```python
from build123d import *

# Parameters (mm, degrees)
ESQUISSE1_R             = 20.5
ESQUISSE1_R_2           = 13
BOSS_EXTRU_1_DEPTH      = 4.5
ENL_V_MAT_EXTRU_1_REACH = 6.5
ESQUISSE2_R             = 1.5
ESQUISSE2_R_2           = 2.11
ENL_V_MAT_EXTRU_2_DEPTH = 2.5


with BuildPart() as part:
    # Esquisse1 → Boss.-Extru.1 (new body)
    with BuildSketch(Plane.XY):
        Circle(ESQUISSE1_R)
        Circle(ESQUISSE1_R_2, mode=Mode.SUBTRACT)
    extrude(amount=BOSS_EXTRU_1_DEPTH)

    # Esquisse2 → Enlèv. mat.-Extru.1 (cut, up to next)
    with BuildSketch(Plane.XY.offset(4.5), mode=Mode.PRIVATE) as enl_v_mat_extru_1_sk1:
        with Locations((0, 17.5)):
            Circle(ESQUISSE2_R)
    enl_v_mat_extru_1_tool1 = extrude(enl_v_mat_extru_1_sk1.sketch, amount=-ENL_V_MAT_EXTRU_1_REACH, mode=Mode.PRIVATE) & part.part
    add(enl_v_mat_extru_1_tool1.solids().sort_by_distance((0, 17.5, 4.5))[0], mode=Mode.SUBTRACT)
    # Esquisse2 → Enlèv. mat.-Extru.1 (cut, up to next)
    with BuildSketch(Plane.XY.offset(4.5), mode=Mode.PRIVATE) as enl_v_mat_extru_1_sk2:
        with Locations((16.25, 0)):
            Circle(ESQUISSE2_R_2)
    enl_v_mat_extru_1_tool2 = extrude(enl_v_mat_extru_1_sk2.sketch, amount=-ENL_V_MAT_EXTRU_1_REACH, mode=Mode.PRIVATE) & part.part
    add(enl_v_mat_extru_1_tool2.solids().sort_by_distance((16.25, 0, 4.5))[0], mode=Mode.SUBTRACT)
    # Esquisse2 → Enlèv. mat.-Extru.1 (cut, up to next)
    with BuildSketch(Plane.XY.offset(4.5), mode=Mode.PRIVATE) as enl_v_mat_extru_1_sk3:
        with Locations((0, -17.5)):
            Circle(ESQUISSE2_R)
    enl_v_mat_extru_1_tool3 = extrude(enl_v_mat_extru_1_sk3.sketch, amount=-ENL_V_MAT_EXTRU_1_REACH, mode=Mode.PRIVATE) & part.part
    add(enl_v_mat_extru_1_tool3.solids().sort_by_distance((0, -17.5, 4.5))[0], mode=Mode.SUBTRACT)
    # Esquisse2 → Enlèv. mat.-Extru.1 (cut, up to next)
    with BuildSketch(Plane.XY.offset(4.5), mode=Mode.PRIVATE) as enl_v_mat_extru_1_sk4:
        with Locations((-16.25, 0)):
            Circle(ESQUISSE2_R_2)
    enl_v_mat_extru_1_tool4 = extrude(enl_v_mat_extru_1_sk4.sketch, amount=-ENL_V_MAT_EXTRU_1_REACH, mode=Mode.PRIVATE) & part.part
    add(enl_v_mat_extru_1_tool4.solids().sort_by_distance((-16.25, 0, 4.5))[0], mode=Mode.SUBTRACT)

    # Esquisse3 → Enlèv. mat.-Extru.2 (cut)
    with BuildSketch(Plane.XY.offset(4.5)):
        with BuildLine():
            Line((-3.25, 17.5), (-3.25, 27.5))
            Line((-3.25, 27.5), (3.25, 27.5))
            Line((3.25, 27.5), (3.25, 17.5))
            ThreePointArc((3.25, 17.5), (0, 14.25), (-3.25, 17.5))
        make_face()
        with BuildLine():
            Line((-3.25, -27.5), (3.25, -27.5))
            Line((3.25, -27.5), (3.25, -17.5))
            ThreePointArc((3.25, -17.5), (0, -14.25), (-3.25, -17.5))
            Line((-3.25, -17.5), (-3.25, -27.5))
        make_face()
    extrude(amount=-ENL_V_MAT_EXTRU_2_DEPTH, mode=Mode.SUBTRACT)


solid = part.part
```
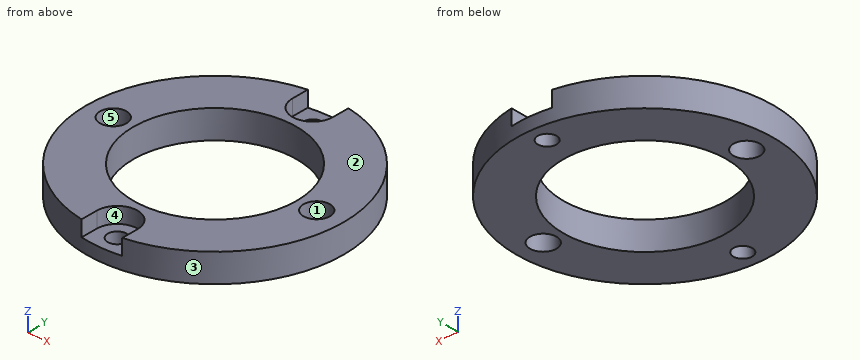
The listing builds one solid part. Answer for the finished solid, in the listing's coordinates (mm). Face numbers are marked on the shaded views. A direction names the side the tool comes from. Give positions to 0.01 mm unless a question says otherwise; leave off trailing zeros. Order: outer loops, then holes, each group sorted by start corner. A loop starts at its lowest first (then second) coordinate and runs counter-clockwise, first axis right, second up.
Item 1: For a pull along X with two mould halves and no side action, classify the marked faces 1, 2 and 3 as pulls with the +X half, pulls with the -X half, needs draft (parallel to the pull), parting line crosses it, or undercut.
From the geometry:
face 1: undercut
face 2: needs draft
face 3: parting line crosses it
Item 2: Find the intervals of material crossed by probe 1 along Y at (x, z) = (0, 1.6); probe 2 along Y at (x, z) = (0, 3.55); probe 3 along Y at (x, z) = (-1, 1.15), in increasing order.
From the geometry:
probe 1: y = -20.5 to -19, -16 to -13, 13 to 16, 19 to 20.5
probe 2: y = -14.25 to -13, 13 to 14.25
probe 3: y = -20.48 to -18.62, -16.38 to -12.96, 12.96 to 16.38, 18.62 to 20.48
Item 3: Which of the six approach directions +Z, -Z, +X, -X, +Y, -Y give full straight-line access (tool end or side, diameter ignored) to the marked faces 4 and 5?
From the geometry:
face 4: +Z, -Y
face 5: +Z, -Z
Item 4: Given pin 1 Ø1.9 at (x, y) = (1, 17) entering from +Z; pin 2 Ø21 at (x, y) = (0, 0) entering from -Z; pin 3 Ø1.2 at (y, z) = (-19.5, 3) entering from -X; pin 4 Ø2 at (x, z) = (-2, 2) entering from +Y, each flat-ended and moving along its own axis, determine where each tip first touches the part or whether it passes through.
From the geometry:
pin 1: stops at z = 2
pin 2: passes through
pin 3: stops at x = -7.94
pin 4: stops at y = 20.48
Item 5: The part is cut by section A-A, the plane x = -16.25. Give the vertices of the cut face in (y, z).
From the geometry:
outline: (-12.5, 0) - (-2.11, 0) - (-2.11, 4.5) - (-12.5, 4.5) - close; (2.11, 0) - (12.5, 0) - (12.5, 4.5) - (2.11, 4.5) - close
Item 6: The part is cut by section B-B, the plane z = 2.7. Give the vertices of the cut face in (x, y).
From the geometry:
outline: (-3.25, -20.24) - (-3.25, -17.5) arc R3.25 cw to (3.25, -17.5) - (3.25, -20.24) arc R20.5 ccw to (3.25, 20.24) - (3.25, 17.5) arc R3.25 cw to (-3.25, 17.5) - (-3.25, 20.24) arc R20.5 ccw to start; hole circle Ø4.22 at (-16.25, 0); hole circle Ø26 at (0, 0); hole circle Ø4.22 at (16.25, 0)
Item 7: The part is cut by section C-C, the plane y = -17. Give the vertices of the cut face in (x, z), and give its area (3 significant figures).
From the geometry:
outline: (-11.46, 0) - (-1.41, 0) - (-1.41, 2) - (-3.21, 2) - (-3.21, 4.5) - (-11.46, 4.5) - close; (1.41, 0) - (11.46, 0) - (11.46, 4.5) - (3.21, 4.5) - (3.21, 2) - (1.41, 2) - close
area: 81.4 mm2
Item 8: The part is cut by section D-D, the plane y = -1. Give the vertices of the cut face in (x, z), and give its area (3 significant figures).
From the geometry:
outline: (-20.48, 0) - (-18.11, 0) - (-18.11, 4.5) - (-20.48, 4.5) - close; (-14.39, 0) - (-12.96, 0) - (-12.96, 4.5) - (-14.39, 4.5) - close; (12.96, 0) - (14.39, 0) - (14.39, 4.5) - (12.96, 4.5) - close; (18.11, 0) - (20.48, 0) - (20.48, 4.5) - (18.11, 4.5) - close
area: 34.2 mm2
